Here's the drawing with two shaded views (mm, measured from the low corner). I have some questions. Coordinates: 2 decimals unless noted, no trailing zeros. Order: outer loops, then holes, each group sorted by start corner. A loop starts at its lowest first (then second) coordinate and runs counter-clockwise, first axis right, second up. Notation, with made-up numbers: M -1,-34 L 54,-34 A8 ccw 54,-19 Z; hole C 58,-20.75 d3. An arc over 180 degrees is marked long. Put each result on its own line as item: value. Start each with the question number.
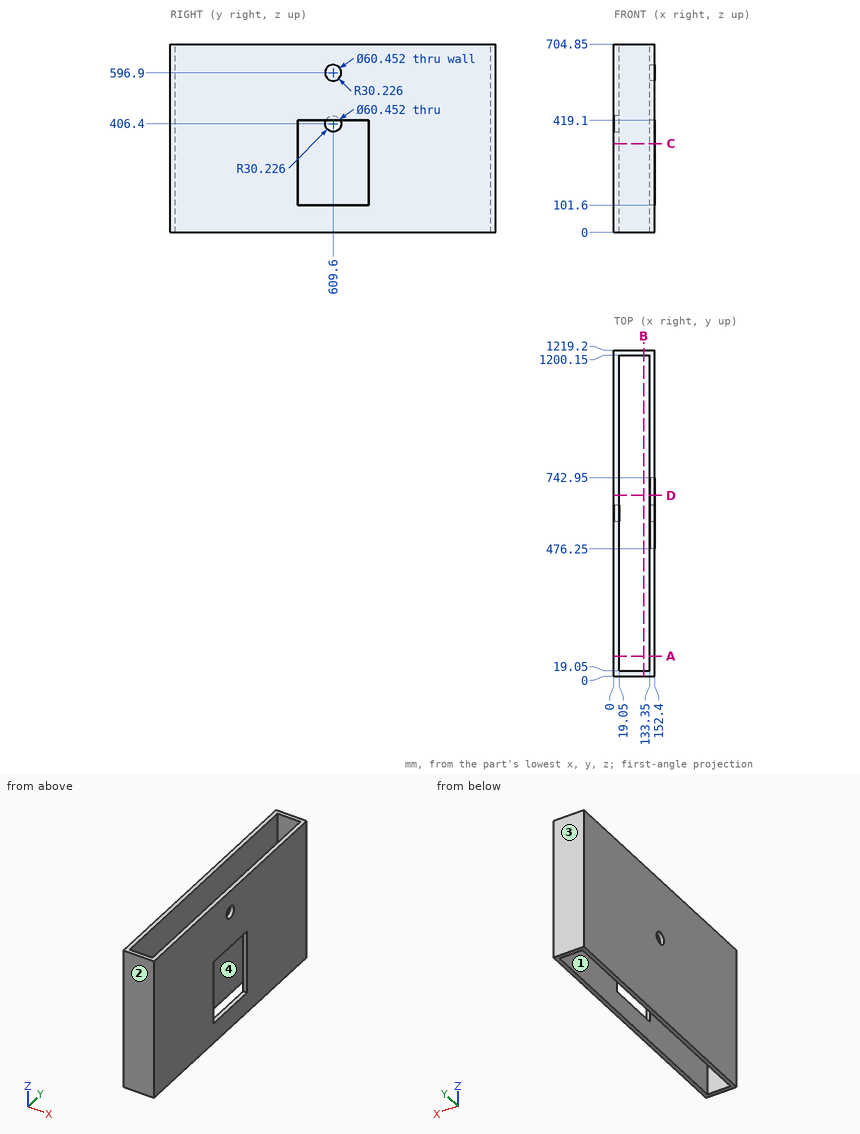
Item 1: If we section it at D-D on y = 676: Write out the boundary of the cut face in (x, z), then the cut area to 3 significant figures.
Item 2: For pin 1 Ø6 at (y, z) = (707, 351.5) entering from +X, with a flat end and sliding along its axis, tell me the tip position at first contact or that it passes through.
Item 3: If we section it at C-C on z = 332: Write out the boundary of the cut face in (x, y).
Item 4: I need wall thicknesses on probe 1 along Z at (x, y) = (138, 609); probe 2 along Y at (x, z) = (137, 596.9); probe 3 along X at (y, z) = (197, 399). Which ranges of each line are inside material? Lowest first, please.
Item 5: If we mould it in two halves opening along Y, with no side actions, what happens to the marked faces 1, 2, 3 and 4? For each: released by +Y, released by -Y, zero draft, split by the parting line, or undercut.
Item 6: If we section it at B-B on x = 111: Write out the boundary of the cut face in (y, z).
Item 7: If we section it at A-A on y = 74: Write out the boundary of the cut face in (x, z).
Geometry check:
1. outline: M 0,0 L 19.05,0 L 19.05,704.85 L 0,704.85 Z; M 133.35,0 L 152.4,0 L 152.4,101.6 L 133.35,101.6 Z; M 133.35,419.1 L 152.4,419.1 L 152.4,704.85 L 133.35,704.85 Z
1. area: 20,800 mm²
2. pin 1: stops at x = 19.05
3. outline: M 0,0 L 152.4,0 L 152.4,476.25 L 133.35,476.25 L 133.35,19.05 L 19.05,19.05 L 19.05,1200.15 L 133.35,1200.15 L 133.35,742.95 L 152.4,742.95 L 152.4,1219.2 L 0,1219.2 Z
4. probe 1: z = 0 to 101.6, 419.1 to 566.68, 627.12 to 704.85
4. probe 2: y = 0 to 579.37, 639.83 to 1219.2
4. probe 3: x = 0 to 19.05, 133.35 to 152.4
5. face 1: undercut
5. face 2: released by -Y
5. face 3: released by +Y
5. face 4: undercut
6. outline: M 0,0 L 19.05,0 L 19.05,704.85 L 0,704.85 Z; M 1200.15,0 L 1219.2,0 L 1219.2,704.85 L 1200.15,704.85 Z
7. outline: M 0,0 L 19.05,0 L 19.05,704.85 L 0,704.85 Z; M 133.35,0 L 152.4,0 L 152.4,704.85 L 133.35,704.85 Z
